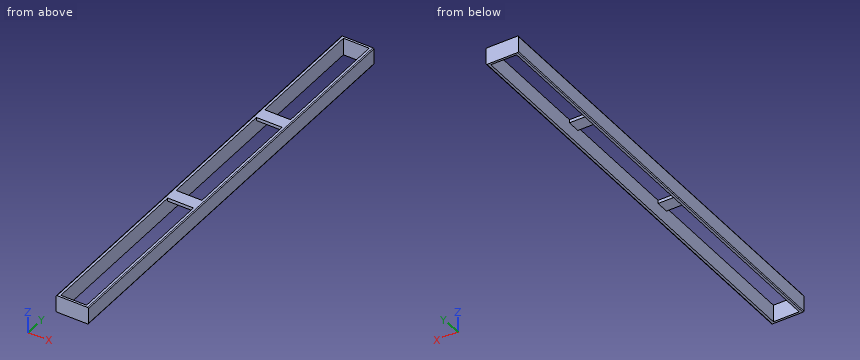
from build123d import *

# Parameters (mm, degrees)
F1_DEPTH = 1020
F2_W     = 60
F2_H     = 382.118
F2_H_2   = 286.796
F2_H_3   = 281.086
F3_DEPTH = 60
F4_DEPTH = 32.5
F5_R     = 2


with BuildPart() as f1:
    # F0 (on Front) → F1 (new body)
    with BuildSketch(Plane.XZ):
        Polygon((30, -20), (37.5, -20), (37.5, 20), (-37.5, 20), (-37.5, -20), (-30, -20), (-30, -12.5), (-30, 12.5), (30, 12.5), (30, -12.5), align=None)
    extrude(amount=F1_DEPTH)

    # F2 (on face) → F3 (cut)
    with BuildSketch(Plane.XY.offset(20)):
        with Locations((0, -823.941)):
            Rectangle(F2_W, F2_H)
        with Locations((0, -459.484)):
            Rectangle(F2_W, F2_H_2)
        with Locations((0, -145.543)):
            Rectangle(F2_W, F2_H_3)
    extrude(amount=-F3_DEPTH, mode=Mode.SUBTRACT)

    # F4 (add): faces of the model
    f4_faces = [f1.faces().sort_by_distance(p)[0] for p in [
        (0, -1017.5, 12.5),
        (0, -2.5, 12.5),
    ]]
    extrude(f4_faces, amount=F4_DEPTH)

    # F5
    f5_edges = [f1.edges().sort_by_distance(p)[0] for p in [
        (-37.5, -510, 20),
        (37.5, -510, 20),
        (-37.5, -510, -20),
        (37.5, -510, -20),
    ]]
    fillet(f5_edges, radius=F5_R)


solid = f1.part
Input: part model. Units: mm. Frame: model coordinates. Give positions to 0.01 mm unless a question says otherwise; leave off trailing zeros. Loops run counter-clockwise (first coordinate to the right, second up) from the corner with the lowest first, then second, coordinate; pieces in that order, holes last. Notation, with made-up numbers: (66.25, 72) -> (72.25, 72) arc R20 ccw to (72.25, 86) -> close; hole circle Ø10 at (76, 88.5). An arc over 180 degrees is marked (long way). Answer as a JSON object with one key per item and string values. Group by question number.
Item 1: Cut plane A-A, the plane y = -779.5. Return the cut outline in (x, z).
Item 2: Line query: probe 1 along Y at (x, z) = (-15.5, 18.5); probe 2 along X at (y, z) = (-901.5, 17); probe 3 along Y at (x, z) = (18.5, -7.5). Output: solid intervals per line, ascending.
Item 3: Cut plane B-B, the plane x = -9.5. Return the cut outline in (y, z).
Item 4: Cut plane C-C, the plane z = -12. Return the cut outline in (x, y).
Item 5: Pin query (flat end, axial travel): P1, Ø4, axis at x = 14, z = 17, coming from the +Y side. Return the tip coordinate at first contact, or that it passes through.
Checks:
{
 "1": {"outline": "(-37.5, -18) arc R2 ccw to (-35.5, -20) -> (-30, -20) -> (-30, 20) -> (-35.5, 20) arc R2 ccw to (-37.5, 18) -> close; (30, -20) -> (35.5, -20) arc R2 ccw to (37.5, -18) -> (37.5, 18) arc R2 ccw to (35.5, 20) -> (30, 20) -> close"},
 "2": {"probe 1": "y = -1020 to -1015, -632.88 to -602.88, -316.09 to -286.09, -5 to 0", "probe 2": "x = -37.5 to -30, 30 to 37.5", "probe 3": "y = -1020 to -1015, -5 to 0"},
 "3": {"outline": "(-1020, -20) -> (-1015, -20) -> (-1015, 20) -> (-1020, 20) -> close; (-632.88, 12.5) -> (-602.88, 12.5) -> (-602.88, 20) -> (-632.88, 20) -> close; (-316.09, 12.5) -> (-286.09, 12.5) -> (-286.09, 20) -> (-316.09, 20) -> close; (-5, -20) -> (0, -20) -> (0, 20) -> (-5, 20) -> close"},
 "4": {"outline": "(-37.5, -1020) -> (37.5, -1020) -> (37.5, 0) -> (-37.5, 0) -> close; hole (-30, -1015) -> (30, -1015) -> (30, -5) -> (-30, -5) -> close"},
 "5": {"P1": "stops at y = 0"}
}
